```python
from build123d import *

# Parameters (mm, degrees)
F0_R     = 11.2
F0_R_2   = 1.75
F0_R_3   = 2.75
F0_R_4   = 4.25
F1_DEPTH = 7


with BuildPart() as f1:
    # F0 (on Top) → F1 (new body)
    with BuildSketch(Plane.XY):
        Polygon((19.521375, 33.261315), (9.893419, 50.243954), (-9.627956, 50.39722), (-19.521375, 33.567845), (-9.893419, 16.585206), (9.627956, 16.43194), align=None)
        with Locations((0, 33.41458)):
            Circle(F0_R, mode=Mode.SUBTRACT)
        with BuildLine():
            ThreePointArc((38.793711, 0.149422), (25.162096, 14.379871), (19.521375, 33.261315))
            Line((19.521375, 33.261315), (9.627956, 16.43194))
            ThreePointArc((9.627956, 16.43194), (9.917718, 5.657179), (19.272335, 0.302687))
            Line((19.272335, 0.302687), (38.793711, 0.149422))
        make_face()
        with Locations((27.107068, 6.250099)):
            Circle(F0_R_2, mode=Mode.SUBTRACT)
        with Locations((22.546168, 11.302348)):
            Circle(F0_R_3, mode=Mode.SUBTRACT)
        with Locations((16.533859, 17.45883)):
            Circle(F0_R_4, mode=Mode.SUBTRACT)
        Polygon((48.421667, -16.833218), (38.793711, 0.149422), (19.272335, 0.302687), (9.378916, -16.526687), (19.006872, -33.509327), (38.528247, -33.662592), align=None)
        with Locations((28.900291, -16.679952)):
            Circle(F0_R, mode=Mode.SUBTRACT)
        with BuildLine():
            Line((-9.893419, 16.585206), (-19.521375, 33.567845))
            ThreePointArc((-19.521375, 33.567845), (-25.029499, 14.647296), (-38.560948, 0.321567))
            Line((-38.560948, 0.321567), (-19.039573, 0.168302))
            ThreePointArc((-19.039573, 0.168302), (-9.853236, 5.806623), (-9.893419, 16.585206))
        make_face()
        with Locations((-23.38672, 5.589327)):
            Circle(F0_R_4, mode=Mode.SUBTRACT)
        with Locations((-21.061205, 13.87438)):
            Circle(F0_R_3, mode=Mode.SUBTRACT)
        with Locations((-18.966278, 20.35036)):
            Circle(F0_R_2, mode=Mode.SUBTRACT)
        Polygon((-19.039573, 0.168302), (-38.560948, 0.321567), (-48.454367, -16.507807), (-38.826411, -33.490447), (-19.305036, -33.643712), (-9.411617, -16.814338), align=None)
        with Locations((-28.932992, -16.661073)):
            Circle(F0_R, mode=Mode.SUBTRACT)
        with BuildLine():
            Line((19.006872, -33.509327), (9.378916, -16.526687))
            ThreePointArc((9.378916, -16.526687), (-0.097182, -11.390247), (-9.411617, -16.814338))
            Line((-9.411617, -16.814338), (-19.305036, -33.643712))
            ThreePointArc((-19.305036, -33.643712), (-0.165298, -28.953612), (19.006872, -33.509327))
        make_face()
        with Locations((-8.14079, -26.600459)):
            Circle(F0_R_2, mode=Mode.SUBTRACT)
        with Locations((-1.484963, -25.176729)):
            Circle(F0_R_3, mode=Mode.SUBTRACT)
        with Locations((6.852861, -23.048157)):
            Circle(F0_R_4, mode=Mode.SUBTRACT)
        with BuildLine():
            ThreePointArc((19.272335, 0.302687), (9.917718, 5.657179), (9.627956, 16.43194))
            Line((9.627956, 16.43194), (-9.893419, 16.585206))
            ThreePointArc((-9.893419, 16.585206), (-9.853236, 5.806623), (-19.039573, 0.168302))
            Line((-19.039573, 0.168302), (-9.411617, -16.814338))
            ThreePointArc((-9.411617, -16.814338), (-0.097182, -11.390247), (9.378916, -16.526687))
            Line((9.378916, -16.526687), (19.272335, 0.302687))
        make_face()
        Circle(F0_R, mode=Mode.SUBTRACT)
    extrude(amount=F1_DEPTH)


solid = f1.part
```
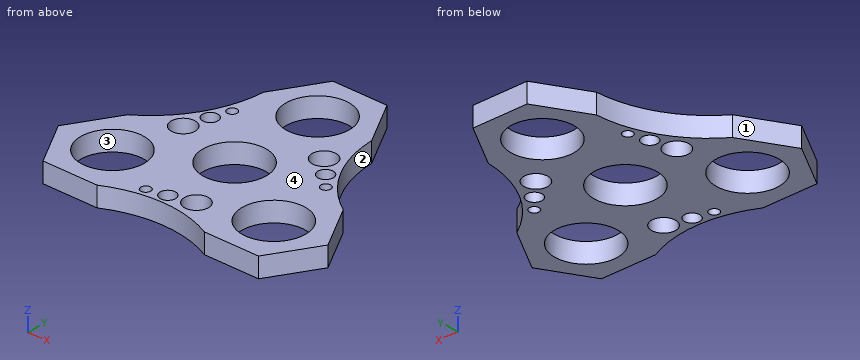
Geometry: final body of the model. Coordinates: model frame, mm. Face numbers are marked on the shaded views. Round coordinates to 2 decimals unless told otherwise and drop trailing zeros. Write each loop counter-clockwise with the first axis right and the second up, starting at its lowest first coordinate (ties: lowest second). Pieces come first, ordered by that corner, then holes.
Item 1: Pin query (flat end, axial travel): P1, Ø4, axis at y = 7, z = 5, coming from the -X side; P2, Ø2, axis at x = 28, z = 3, coming from the +Y side; P3, Ø1.5, axis at y = 30, z = 5, coming from the +X side. Return the tip coordinate at first contact, or that it passes through.
Item 2: Section query B-B (z = 3). Give the number of separate pieces and of enclosed holes in the cut face, plus the area to 3 significant figures.
Item 3: Section query C-C (y = -4). Return loops of the section in (x, z), plus the area to 3 significant figures.
Item 4: Mould query, pull axis X, two halves, no side actions, for the marked faces 1, 2, 3 and 4. Classes: +X half, -X half, draft (parallel to the pull), parting line (faces both ways), or undercut.
Item 5: Section query A-A (x = 0). Return loops of the section in (y, z), plus the area to 3 significant figures.
Item 6: Material intervals for L1, parallel to Y at x = -25, z = 6.5; L2, parallel to Y at x = -27, z = 4.75; L3, parallel to Y at x = -8.5, z = 5.25, sorted ascending.
Completed:
1. P1: stops at x = -32.62
1. P2: stops at y = 11.5
1. P3: stops at x = 19.93
2. separate pieces: 1
2. enclosed holes: 13
2. area: 3,170 mm2
3. outline: (-41.1, 0) - (-10.46, 0) - (-10.46, 7) - (-41.1, 7) - close; (10.46, 0) - (41.15, 0) - (41.15, 7) - (10.46, 7) - close
3. area: 429 mm2
4. face 1: -X half
4. face 2: +X half
4. face 3: undercut
4. face 4: draft
5. outline: (-28.95, 0) - (-27.49, 0) - (-27.49, 7) - (-28.95, 7) - close; (-22.86, 0) - (-11.2, 0) - (-11.2, 7) - (-22.86, 7) - close; (11.2, 0) - (22.21, 0) - (22.21, 7) - (11.2, 7) - close; (44.61, 0) - (50.32, 0) - (50.32, 7) - (44.61, 7) - close
5. area: 209 mm2
6. L1: y = -33.6 to -27.15, -6.17 to 1.66, 9.52 to 14.7
6. L2: y = -33.58 to -27.69, -5.63 to 3.35, 7.83 to 11.53
6. L3: y = -29.82 to -28.31, -24.89 to -7.29, 7.29 to 26.12, 40.71 to 50.39
